The model under review builds one solid part; all positions refer to its coordinate system, in mm. Coordinates: 2 decimals unless noted, no trailing zeros. Loops run counter-clockwise (first coordinate to the right, second up) from the corner with the lowest first, then second, coordinate; pieces in that order, holes last. Notation, with made-up numbers: M 59.25,73 L 91.25,73 A26 cw 91.25,111 Z; hole C 18.25,18.25 d3. An arc over 180 degrees is marked long. One line per item, written item: value.
```python
from build123d import *

# Parameters (mm, degrees)
LM12UU_0_INT_R          = 6
LM12UU_0_INT_DEPTH      = 34
LM12UU_0_INT_ROLL_ANGLE = -90
LM12UU_0_EXT_R          = 11
LM12UU_0_EXT_DEPTH      = 32
LM12UU_0_EXT_ROLL_ANGLE = -90


with BuildPart() as lm12uu_0_int:
    # lm12uu_0_int → lm12uu_0_int (new body)
    with BuildSketch(Plane.XY):
        Circle(LM12UU_0_INT_R)
    extrude(amount=LM12UU_0_INT_DEPTH)


with BuildPart() as lm12uu_0_int_1:
    # lm12uu_0_int roll: moved
    add(lm12uu_0_int.part.rotate(Axis((0, 0, 0), (1, 0, 0)), LM12UU_0_INT_ROLL_ANGLE))


with BuildPart() as lm12uu_0_int_2:
    # lm12uu_0_int placement: moved
    add(lm12uu_0_int_1.part.moved(Location((0, -82.2, 0))))


with BuildPart() as lm12uu_0_body:
    # lm12uu_0_ext → lm12uu_0_ext (new body)
    with BuildSketch(Plane.XY):
        Circle(LM12UU_0_EXT_R)
    extrude(amount=LM12UU_0_EXT_DEPTH)


with BuildPart() as lm12uu_0_body_1:
    # lm12uu_0_ext roll: moved
    add(lm12uu_0_body.part.rotate(Axis((0, 0, 0), (1, 0, 0)), LM12UU_0_EXT_ROLL_ANGLE))


with BuildPart() as lm12uu_0_body_2:
    # lm12uu_0_ext placement: moved
    add(lm12uu_0_body_1.part.moved(Location((0, -81.2, 0))))

    # lm12uu_0: cut lm12uu_0_int
    add(lm12uu_0_int_2.part, mode=Mode.SUBTRACT)


solid = lm12uu_0_body_2.part
```
(1) Add section D-D on x = 7.5. State the section outline as (y, z) points, then the cut area to 3 significant figures.
Checks:
outline: M -81.2,-8.05 L -49.2,-8.05 L -49.2,8.05 L -81.2,8.05 Z
area: 515 mm^2
(2) Insertion check: pin 1 Ø8 at (x, y) = (4.5, -72.5) entering from -Z; pin 2 Ø1.5 at (y, z) = (-53.5, 7) entering from +X; pin 3 Ø4 at (x, y) = (-5, -61.5) entering from -Z. Each pin has a flat end and moves straight along its axis. Give the tip position at first contact, or say it passes through.
Checks:
pin 1: z = -10.99
pin 2: x = 9.05
pin 3: z = -10.58
(3) To check wall thickness, follow L1, parallel to Z at x = 0, y = -63.5; L2, parallel to X at y = -62, z = -3.5; L3, parallel to Z at x = -1, y = -69. State the ranges of each line that lie inside material, in increasing order. Write a range as [from, to].
Checks:
L1: [-11, -6], [6, 11]
L2: [-10.43, -4.87], [4.87, 10.43]
L3: [-10.95, -5.92], [5.92, 10.95]
(4) Add section C-C on y = -51. State the section outline as (x, z) points.
Checks:
outline: C 0,0 d22; hole C 0,0 d12
(5) Add section A-A on x = 0. State the section outline as (y, z) points, then the cut area to 3 significant figures.
Checks:
outline: M -81.2,-11 L -49.2,-11 L -49.2,-6 L -81.2,-6 Z; M -81.2,6 L -49.2,6 L -49.2,11 L -81.2,11 Z
area: 320 mm^2
(6) Add section B-B on z = 0. State the section outline as (x, y) points.
Checks:
outline: M -11,-81.2 L -6,-81.2 L -6,-49.2 L -11,-49.2 Z; M 6,-81.2 L 11,-81.2 L 11,-49.2 L 6,-49.2 Z
